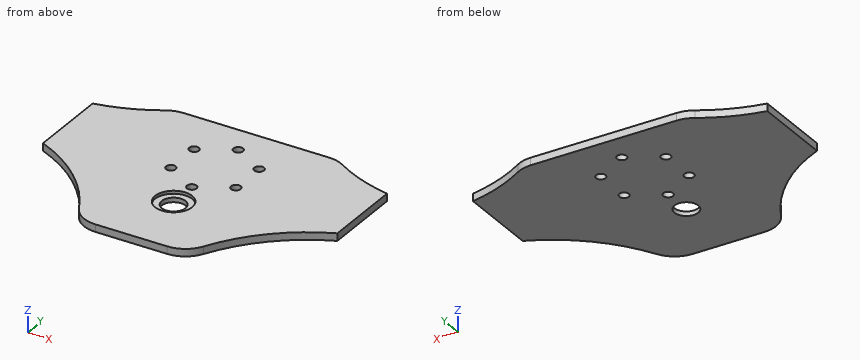
from build123d import *

# Parameters (mm, degrees)
ESBO_O1_R                = 3.25
ESBO_O1_R_2              = 8
RESSALTO_EXTRUS_O1_DEPTH = 5
ESBO_O2_R                = 12.5
ESBO_O2_R_2              = 8
CORTE_EXTRUS_O1_DEPTH    = 2


with BuildPart() as part:
    # Esboço1 → Ressalto-extrusão1 (new body)
    with BuildSketch(Plane.XY):
        with BuildLine():
            Line((-49.119135606, 68), (49.119135606, 68))
            ThreePointArc((49.119135606, 68), (54.543435225, 67.250375935), (59.56111629, 65.057697365))
            ThreePointArc((59.56111629, 65.057697365), (78.583692726, 55.703629757), (99, 50))
            Line((99, 50), (99, -4))
            ThreePointArc((99, -4), (65.800143376, -25.584477196), (41.890064111, -57.150728877))
            ThreePointArc((41.890064111, -57.150728877), (34.522230169, -65.073584532), (24.106246719, -68))
            Line((24.106246719, -68), (-24.106246719, -68))
            ThreePointArc((-24.106246719, -68), (-34.522230169, -65.073584532), (-41.890064111, -57.150728877))
            ThreePointArc((-41.890064111, -57.150728877), (-65.800143376, -25.584477196), (-99, -4))
            Line((-99, -4), (-99, 50))
            ThreePointArc((-99, 50), (-78.583692726, 55.703629757), (-59.56111629, 65.057697365))
            ThreePointArc((-59.56111629, 65.057697365), (-54.543435225, 67.250375935), (-49.119135606, 68))
        make_face()
        with Locations((0, 48.25)):
            Circle(ESBO_O1_R, mode=Mode.SUBTRACT)
        with Locations((21.867141446, 35.625)):
            Circle(ESBO_O1_R, mode=Mode.SUBTRACT)
        with Locations((21.867141446, 10.375)):
            Circle(ESBO_O1_R, mode=Mode.SUBTRACT)
        with Locations((0, -2.25)):
            Circle(ESBO_O1_R, mode=Mode.SUBTRACT)
        with Locations((-21.867141446, 10.375)):
            Circle(ESBO_O1_R, mode=Mode.SUBTRACT)
        with Locations((-21.867141446, 35.625)):
            Circle(ESBO_O1_R, mode=Mode.SUBTRACT)
        with Locations((0, -22)):
            Circle(ESBO_O1_R_2, mode=Mode.SUBTRACT)
    extrude(amount=RESSALTO_EXTRUS_O1_DEPTH)

    # Esboço2 → Corte-extrusão1 (cut)
    with BuildSketch(Plane.XY.offset(5)):
        with Locations((0, -22)):
            Circle(ESBO_O2_R)
        with Locations((0, -22)):
            Circle(ESBO_O2_R_2, mode=Mode.SUBTRACT)
    extrude(amount=-CORTE_EXTRUS_O1_DEPTH, mode=Mode.SUBTRACT)


solid = part.part
Can you work these out from the model? Positions are in its coordinate system, mm. Coordinates: 2 decimals unless noted, no trailing zeros. Write each loop counter-clockwise with the first axis right and the second up, starting at its lowest first coordinate (ties: lowest second). Pieces come first, ordered by that corner, then holes. Notation, with made-up numbers: (-36, 26) -> (-28, 26) arc R26 cw to (-28, 59) -> close; hole circle Ø7 at (-34, 16). An arc over 180 degrees is marked (long way). Answer as CSV lines item,"result".
1) If we section it at D-D on y = -7.5: Please give me the cut outline in (x, z), then the cut area to 3 significant figures.
Check result:
outline,"(-91.55, 0) -> (91.55, 0) -> (91.55, 5) -> (-91.55, 5) -> close"
area,"916 mm²"
2) If we section it at B-B on z = 1.8: Count the separate pieces of the cut face and the enclosed holes in it, then the cut area to 3 significant figures.
Check result:
separate pieces,"1"
enclosed holes,"7"
area,"20,500 mm²"
3) Will this pin go through, and if not, where does the flat tip stop? P1, Ø2, axis at y = -22, z = 2.5, coming from the +X side.
Check result:
P1,"x = 71.04"
4) If we section it at C-C on x = 66: Please give me the cut outline in (y, z), then the cut area to 3 significant figures.
Check result:
outline,"(-25.4, 0) -> (61.4, 0) -> (61.4, 5) -> (-25.4, 5) -> close"
area,"434 mm²"
5) If we section it at A-A on x = 0: Please give me the cut outline in (y, z), then the cut area to 3 significant figures.
Check result:
outline,"(-68, 0) -> (-30, 0) -> (-30, 3) -> (-34.5, 3) -> (-34.5, 5) -> (-68, 5) -> close; (-14, 0) -> (-5.5, 0) -> (-5.5, 5) -> (-9.5, 5) -> (-9.5, 3) -> (-14, 3) -> close; (1, 0) -> (45, 0) -> (45, 5) -> (1, 5) -> close; (51.5, 0) -> (68, 0) -> (68, 5) -> (51.5, 5) -> close"
area,"517 mm²"
6) If I drill on line 1 (Y direction, x = 0, z = 1.1); line 2 (Y direction, x = 0, z = 3.75); line 3 (Z direction, x = -9.5, y = -24), over which ranges is the centre line in solid material (lowest first)? Write a range as from..to.
Check result:
line 1,"-68..-30, -14..-5.5, 1..45, 51.5..68"
line 2,"-68..-34.5, -9.5..-5.5, 1..45, 51.5..68"
line 3,"0..3"
